Geometry check sheet. Reference: the model listing, model coordinates, mm. Face numbers are marked on the shaded views. A direction names the side the tool comes from. Coordinates: 2 decimals unless noted, no trailing zeros. Loops run counter-clockwise (first coordinate to the right, second up) from the corner with the lowest first, then second, coordinate; pieces in that order, holes last.
from build123d import *

# Parameters (mm, degrees)
SKETCH_1_R           = 21.4
EXTRUDE_2_DEPTH      = 0.5
SKETCH_6_R           = 19.2
SHELL_1_T            = -3
SKETCH_7_R           = 2.5
CUT_EXTRUDE_1_DEPTH  = 32.720182984
SKETCH_8_R           = 7.8
CUT_EXTRUDE_2_DEPTH  = 1.4
CHAMFER_1_SIZE       = 0.5
CUT_EXTRUDE_11_DEPTH = 7
HOLE_WIZARD_M3_1_D   = 2.5


with BuildPart() as part:
    # 草图1 → 凸台-拉伸2 (new body)
    with BuildSketch(Plane(origin=(0, 0, 0), x_dir=(1, 0, 0), z_dir=(0, 1, 0))):
        with Locations(Location((0, 0, 0), (0, 0, 270))):
            Circle(SKETCH_1_R)
    extrude(amount=EXTRUDE_2_DEPTH)

    # 草图6 → section 0 of loft_1
    with BuildSketch(Plane(origin=(0, 9.5, 0), x_dir=(1, 0, 0), z_dir=(0, 1, 0)), mode=Mode.PRIVATE) as loft_1_s0:
        Circle(SKETCH_6_R)
    # loft up to a face of the part (loft_1)
    loft([loft_1_s0.sketch, part.faces().sort_by_distance((0, 0.5, 0))[0]])

    # 抽壳1
    shell_1_openings = [part.faces().sort_by_distance(p)[0] for p in [
        (0, 0, 0),
    ]]
    offset(amount=SHELL_1_T, openings=shell_1_openings)

    # 草图7 → 切除-拉伸1 (cut, through all)
    with BuildSketch(Plane(origin=(0, 9.5, 0), x_dir=(1, 0, 0), z_dir=(0, 1, 0))):
        with Locations(Location((0, 0, 0), (0, 0, 270))):
            Circle(SKETCH_7_R)
    extrude(amount=-CUT_EXTRUDE_1_DEPTH, mode=Mode.SUBTRACT)

    # 草图8 → 切除-拉伸2 (cut)
    with BuildSketch(Plane(origin=(0, 9.5, 0), x_dir=(1, 0, 0), z_dir=(0, 1, 0))):
        with Locations(Location((0, 0, 0), (0, 0, 270))):
            Circle(SKETCH_8_R)
    extrude(amount=-CUT_EXTRUDE_2_DEPTH, mode=Mode.SUBTRACT)

    # 倒角1
    chamfer_1_edges = [part.edges().sort_by_distance(p)[0] for p in [
        (0, 9.5, -7.8),
        (0, 8.1, -7.8),
    ]]
    chamfer(chamfer_1_edges, length=CHAMFER_1_SIZE)

    # 草图9 → 切除-拉伸11 (cut)
    with BuildSketch(Plane(origin=(0, 9.5, 0), x_dir=(1, 0, 0), z_dir=(0, 1, 0))):
        with BuildLine():
            Line((-2, 15.451390353), (-2, 20.653389552))
            ThreePointArc((-2, 20.653389552), (0, 20.75), (2, 20.653389552))
            Line((2, 20.653389552), (2, 15.451390353))
            ThreePointArc((2, 15.451390353), (0, 13.451390353), (-2, 15.451390353))
        make_face()
        with BuildLine():
            Line((2.601690797, 11.507097509), (5.981760612, 19.869097614))
            ThreePointArc((5.981760612, 19.869097614), (7.869025388, 19.200024465), (9.683013266, 18.352159385))
            Line((9.683013266, 18.352159385), (6.310179323, 10.008060201))
            ThreePointArc((6.310179323, 10.008060201), (3.706416406, 8.903334592), (2.601690797, 11.507097509))
        make_face()
        with BuildLine():
            Line((-2.601690797, 11.507097509), (-5.981760612, 19.869097614))
            ThreePointArc((-5.981760612, 19.869097614), (-7.869025388, 19.200024465), (-9.683013266, 18.352159385))
            Line((-9.683013266, 18.352159385), (-6.310179323, 10.008060201))
            ThreePointArc((-6.310179323, 10.008060201), (-3.706416406, 8.903334592), (-2.601690797, 11.507097509))
        make_face()
        with BuildLine():
            Line((15.451390353, 2), (20.653389552, 2))
            ThreePointArc((20.653389552, 2), (20.75, 0), (20.653389552, -2))
            Line((20.653389552, -2), (15.451390353, -2))
            ThreePointArc((15.451390353, -2), (13.451390353, 0), (15.451390353, 2))
        make_face()
        with BuildLine():
            Line((11.507097509, 2.601690797), (19.869097614, 5.981760612))
            ThreePointArc((19.869097614, 5.981760612), (19.200024465, 7.869025388), (18.352159385, 9.683013266))
            Line((18.352159385, 9.683013266), (10.008060201, 6.310179323))
            ThreePointArc((10.008060201, 6.310179323), (8.903334592, 3.706416406), (11.507097509, 2.601690797))
        make_face()
        with BuildLine():
            Line((11.507097509, -2.601690797), (19.869097614, -5.981760612))
            ThreePointArc((19.869097614, -5.981760612), (19.200024465, -7.869025388), (18.352159385, -9.683013266))
            Line((18.352159385, -9.683013266), (10.008060201, -6.310179323))
            ThreePointArc((10.008060201, -6.310179323), (8.903334592, -3.706416406), (11.507097509, -2.601690797))
        make_face()
        with BuildLine():
            Line((2, -15.451390353), (2, -20.653389552))
            ThreePointArc((2, -20.653389552), (0, -20.75), (-2, -20.653389552))
            Line((-2, -20.653389552), (-2, -15.451390353))
            ThreePointArc((-2, -15.451390353), (0, -13.451390353), (2, -15.451390353))
        make_face()
        with BuildLine():
            Line((2.601690797, -11.507097509), (5.981760612, -19.869097614))
            ThreePointArc((5.981760612, -19.869097614), (7.869025388, -19.200024465), (9.683013266, -18.352159385))
            Line((9.683013266, -18.352159385), (6.310179323, -10.008060201))
            ThreePointArc((6.310179323, -10.008060201), (3.706416406, -8.903334592), (2.601690797, -11.507097509))
        make_face()
        with BuildLine():
            Line((-2.601690797, -11.507097509), (-5.981760612, -19.869097614))
            ThreePointArc((-5.981760612, -19.869097614), (-7.869025388, -19.200024465), (-9.683013266, -18.352159385))
            Line((-9.683013266, -18.352159385), (-6.310179323, -10.008060201))
            ThreePointArc((-6.310179323, -10.008060201), (-3.706416406, -8.903334592), (-2.601690797, -11.507097509))
        make_face()
        with BuildLine():
            Line((-15.451390353, -2), (-20.653389552, -2))
            ThreePointArc((-20.653389552, -2), (-20.75, 0), (-20.653389552, 2))
            Line((-20.653389552, 2), (-15.451390353, 2))
            ThreePointArc((-15.451390353, 2), (-13.451390353, 0), (-15.451390353, -2))
        make_face()
        with BuildLine():
            Line((-11.507097509, -2.601690797), (-19.869097614, -5.981760612))
            ThreePointArc((-19.869097614, -5.981760612), (-19.200024465, -7.869025388), (-18.352159385, -9.683013266))
            Line((-18.352159385, -9.683013266), (-10.008060201, -6.310179323))
            ThreePointArc((-10.008060201, -6.310179323), (-8.903334592, -3.706416406), (-11.507097509, -2.601690797))
        make_face()
        with BuildLine():
            Line((-11.507097509, 2.601690797), (-19.869097614, 5.981760612))
            ThreePointArc((-19.869097614, 5.981760612), (-19.200024465, 7.869025388), (-18.352159385, 9.683013266))
            Line((-18.352159385, 9.683013266), (-10.008060201, 6.310179323))
            ThreePointArc((-10.008060201, 6.310179323), (-8.903334592, 3.706416406), (-11.507097509, 2.601690797))
        make_face()
    extrude(amount=-CUT_EXTRUDE_11_DEPTH, mode=Mode.SUBTRACT)

    # M3 螺纹孔的螺纹孔钻头1 (through all)
    with Locations(Plane(origin=(-8.838834765, 9.5, 8.838834765), x_dir=(0, 0, 1), z_dir=(0, 1, 0))):
        with Locations((0, 0), (0, 17.67766953), (-17.67766953, 17.67766953), (-17.67766953, 0)):
            Hole(HOLE_WIZARD_M3_1_D / 2)


solid = part.part
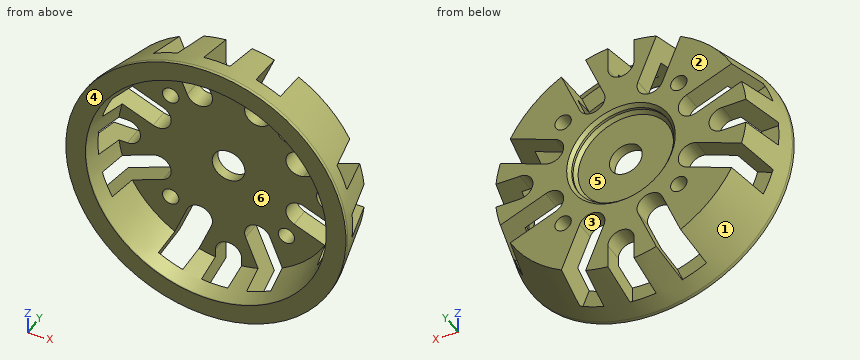
(1) Access from +Z, -Z, +X, -X, +Y, -Y to the whole of each face (thin tool, end or side, straight path). Record for the marked faces 4, 5 and 6.
Findings:
face 4: +Z, -Z, +X, -X, -Y
face 5: +Y
face 6: -Y
(2) Scan lines: L1, parallel to X at y = 8.5, z = -12; L2, parallel to Z at x = -12, y = 8; L3, parallel to X at y = 4, z = 17.5. Record each from-to range of solid material in increasing order.
Findings:
L1: x = -15.3 to -7.12, -2.8 to 2.8, 7.12 to 15.3
L2: z = -15.45 to -7.12, -2.8 to 2.8, 7.12 to 15.45
L3: x = -10.76 to -9.34, -5.02 to -2, 2 to 5.02, 9.34 to 10.76
(3) Draft check along Z on the marked faces 1, 2 and 3. Enter one of: +Z half, -Z half, draft (parallel to the pull), parting line (faces both ways), or undercut.
Findings:
face 1: parting line
face 2: draft
face 3: undercut
(4) Gauge pin test, flat ends, axial feed: pin 1 Ø2.5 at (y, z) = (4.5, 17) entering from +X; pin 2 Ø20.5 at (x, z) = (0, 0) entering from -Y; pin 3 Ø1 at (x, z) = (-2, 2) entering from +Y. Record the tip position at first contact, or that the pin passes through.
Findings:
pin 1: stops at x = 13.07
pin 2: stops at y = 6.5
pin 3: stops at y = 8.1
(5) Sectioned sample at A-A on x = 0. State how many separate pieces and enclosed holes the cut face has, and give its area (3 significant figures).
Findings:
separate pieces: 4
enclosed holes: 0
area: 66.4 mm2
(6) Sectioned sample at D-D on y = 1.75. Record the cut outline in (x, z), and give its area (3 significant figures).
Findings:
outline: circle Ø42.19 at (0, 0); hole circle Ø36.01 at (0, 0)
area: 379 mm2
